```python
from build123d import *

# Parameters (mm, degrees)
SKETCH1_R           = 62.811183182
SKETCH1_R_2         = 3.25
SKETCH1_R_3         = 36.5175
BOSS_EXTRUDE1_DEPTH = 10
BOSS_EXTRUDE2_START = -100
SKETCH1_3_R         = 62.811183182
BOSS_EXTRUDE2_DEPTH = 100


with BuildPart() as part:
    # Sketch1 → Boss-Extrude1 (new body)
    # profile 1 of 2: a face of its own
    with BuildSketch(Plane(origin=(0, 0, 0), x_dir=(0, 0, -1), z_dir=(1, 0, 0))):
        Circle(SKETCH1_R)
        with BuildLine():
            ThreePointArc((43, 34.9), (40.627564928, 40.627564928), (34.9, 43))
            Line((34.9, 43), (-34.9, 43))
            ThreePointArc((-34.9, 43), (-40.627564928, 40.627564928), (-43, 34.9))
            Line((-43, 34.9), (-43, -34.9))
            ThreePointArc((-43, -34.9), (-40.627564928, -40.627564928), (-34.9, -43))
            Line((-34.9, -43), (34.9, -43))
            ThreePointArc((34.9, -43), (40.627564928, -40.627564928), (43, -34.9))
            Line((43, -34.9), (43, 34.9))
        make_face(mode=Mode.SUBTRACT)
    # profile 2 of 2: a face of its own
    with BuildSketch(Plane(origin=(0, 0, 0), x_dir=(0, 0, -1), z_dir=(1, 0, 0))):
        with BuildLine():
            Line((43, -34.9), (43, 34.9))
            ThreePointArc((43, 34.9), (40.627564928, 40.627564928), (34.9, 43))
            Line((34.9, 43), (-34.9, 43))
            ThreePointArc((-34.9, 43), (-40.627564928, 40.627564928), (-43, 34.9))
            Line((-43, 34.9), (-43, -34.9))
            ThreePointArc((-43, -34.9), (-40.627564928, -40.627564928), (-34.9, -43))
            Line((-34.9, -43), (34.9, -43))
            ThreePointArc((34.9, -43), (40.627564928, -40.627564928), (43, -34.9))
        make_face()
        with Locations((-34.9, -34.9)):
            Circle(SKETCH1_R_2, mode=Mode.SUBTRACT)
        with Locations((34.9, -34.9)):
            Circle(SKETCH1_R_2, mode=Mode.SUBTRACT)
        with Locations((34.9, 34.9)):
            Circle(SKETCH1_R_2, mode=Mode.SUBTRACT)
        with Locations((-34.9, 34.9)):
            Circle(SKETCH1_R_2, mode=Mode.SUBTRACT)
        Circle(SKETCH1_R_3, mode=Mode.SUBTRACT)
    extrude(amount=BOSS_EXTRUDE1_DEPTH)

    # Sketch1_3 → Boss-Extrude2 (add)
    with BuildSketch(Plane(origin=(0, 0, 0), x_dir=(0, 0, -1), z_dir=(1, 0, 0)).offset(BOSS_EXTRUDE2_START)):
        Circle(SKETCH1_3_R)
        with BuildLine():
            ThreePointArc((43, 34.9), (40.627564928, 40.627564928), (34.9, 43))
            Line((34.9, 43), (-34.9, 43))
            ThreePointArc((-34.9, 43), (-40.627564928, 40.627564928), (-43, 34.9))
            Line((-43, 34.9), (-43, -34.9))
            ThreePointArc((-43, -34.9), (-40.627564928, -40.627564928), (-34.9, -43))
            Line((-34.9, -43), (34.9, -43))
            ThreePointArc((34.9, -43), (40.627564928, -40.627564928), (43, -34.9))
            Line((43, -34.9), (43, 34.9))
        make_face(mode=Mode.SUBTRACT)
    extrude(amount=BOSS_EXTRUDE2_DEPTH)


solid = part.part
```
Work out the finished part from the listing and answer in its coordinate system (mm). A direction names the side the tool comes from. Give positions to 0.01 mm unless a question says otherwise; leave off trailing zeros. Write each loop counter-clockwise with the first axis right and the second up, starting at its lowest first coordinate (ties: lowest second). Pieces come first, ordered by that corner, then holes. Notation, with made-up numbers: (18, 69) - (72, 69) arc R30 ccw to (72, 105) - close; hole circle Ø6 at (84, 44). An arc over 180 degrees is marked (long way). Use one line per item in the form item = value.
1. Determine the mould class of faces 1 (the face through (-100, -46, -4)), 2 (the face through (-45.77, 62.277, 8.177)), 3 (the face through (4.93, -35.65, 7.92)) for opening direction Y: released by +Y, released by -Y, zero draft, split by the parting line, or undercut.
Filled in:
face_1 = zero draft
face_2 = split by the parting line
face_3 = undercut
2. A cutting plane is placed at D-D (y = 49). Write down the section's boundary in (x, z), and give its area (3 significant figures).
Filled in:
outline = (-100, -39.3) - (10, -39.3) - (10, 39.3) - (-100, 39.3) - close
area = 8,650 mm^2
3. Each of these flat-tipped pins is pushed along its axis until it touches: pin 1 Ø6 at (y, z) = (-34.9, 34.9) entering from +X; pin 2 Ø6 at (x, z) = (-68, -5) entering from -Y; pin 3 Ø2 at (x, y) = (-21, 28.5) entering from +Z; pin 4 Ø10 at (x, z) = (-55.5, -33) entering from +Y. Where does it stop, or does it pass through?
Filled in:
pin_1 = through
pin_2 = -62.78
pin_3 = 56.47
pin_4 = 56.22
4. A cutting plane is placed at C-C (x = -84). Write down the section's boundary in (y, z).
Filled in:
outline = circle Ø125.62 at (0, 0); hole (-43, -34.9) arc R8.1 ccw to (-34.9, -43) - (34.9, -43) arc R8.1 ccw to (43, -34.9) - (43, 34.9) arc R8.1 ccw to (34.9, 43) - (-34.9, 43) arc R8.1 ccw to (-43, 34.9) - close
5. Consider L1, parallel to Y at x = -17, z = 1.5; L2, parallel to Z at x = -41, y = -2; L3, parallel to Y at x = 5, z = 0. Determine where each line is inside the solid, lowest interval first.
Filled in:
L1 = -62.79 to -43, 43 to 62.79
L2 = -62.78 to -43, 43 to 62.78
L3 = -62.81 to -36.52, 36.52 to 62.81
6. For faces 4 (the face through (4.93, 35.043, 38.147)), 5 (the face through (-51, 0, 43)), determine the directions among +Z, -Z, +X, -X, +Y, -Y from which every point of the face is accessible in a straight line to the end or side of a thin tool.
Filled in:
face_4 = +X, -X
face_5 = -X
7. A cutting plane is placed at A-A (z = 0). Write down the section's boundary in (x, y), and give its area (3 significant figures).
Filled in:
outline = (-100, -62.81) - (10, -62.81) - (10, -36.52) - (0, -36.52) - (0, -43) - (-100, -43) - close; (-100, 43) - (0, 43) - (0, 36.52) - (10, 36.52) - (10, 62.81) - (-100, 62.81) - close
area = 4,490 mm^2
